Geometry check sheet. Reference: drawing and pictorial views, mm from the part's lowest x, y, z. Coordinates: 2 decimals unless noted, no trailing zeros. Write each loop counter-clockwise with the first axis right and the second up, starting at its lowest first coordinate (ties: lowest second). Pieces come first, ordered by that corner, then holes. Notation, with made-up numbers: (-28.5, 3.5) - (-14.5, 3.5) arc R21 ccw to (-14.5, 26.5) - close; hole circle Ø9 at (36, 77). An arc over 180 degrees is marked (long way). Use one line per item in the form item = value. Start each with the question number.
(1) Sectioned sample at B-B (x = 58.42). Record the cut outline in (y, z).
(2) Sectioned sample at A-A (y = 6.35). Record the cut outline in (x, z) (3 decimals).
(3) Material ranges on line 1 (Z direction, x = 12.7, y = 9) (3 decimals); line 2 (Y direction, x = 58.42, z = 9.5); line 3 (X direction, y = 7.25, z = 13), recorded low to high. Write a range as [from, to].
(4) Mould release check, pull along X, two halves, no side actions. Record for the marked faces 1, 2, 3 and 4: released by +X, released by -X, zero draft, split by the parting line, or undercut.
(5) Sectioned sample at C-C (z = 15.75). Record the cut outline in (x, y).
(6) Gauge pin test, flat end, axial feed: pin 1 Ø1 at (x, z) = (46.5, 16) entering from -Y. Record the tip position at first contact, or that the pin passes through.
(7) Sectioned sample at D-D (y = 1). Record the cut outline in (x, z) (3 decimals).
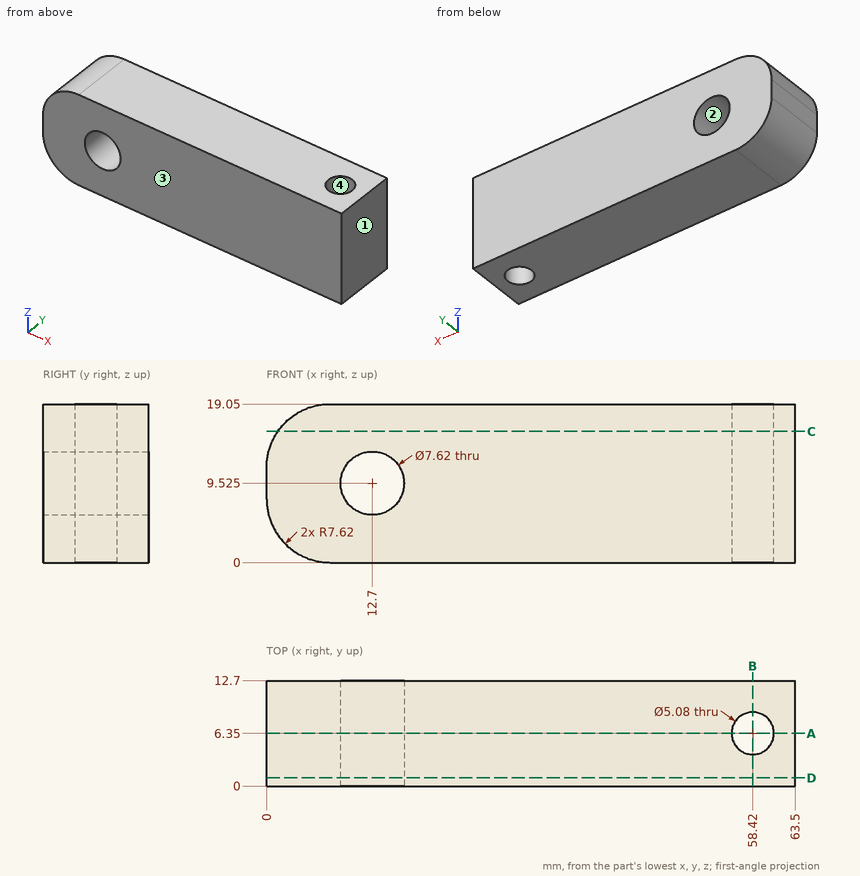
Answers below:
q1.outline = (0, 0) - (3.81, 0) - (3.81, 19.05) - (0, 19.05) - close; (8.89, 0) - (12.7, 0) - (12.7, 19.05) - (8.89, 19.05) - close
q2.outline = (0, 7.62) arc R7.62 ccw to (7.62, 0) - (55.88, 0) - (55.88, 19.05) - (7.62, 19.05) arc R7.62 ccw to (0, 11.43) - close; (60.96, 0) - (63.5, 0) - (63.5, 19.05) - (60.96, 19.05) - close; hole circle Ø7.62 at (12.7, 9.525)
q3.line_1 = [0, 5.715], [13.335, 19.05]
q3.line_2 = [0, 3.81], [8.89, 12.7]
q3.line_3 = [0.16, 11.14], [14.26, 56.04], [60.8, 63.5]
q4.face_1 = released by +X
q4.face_2 = undercut
q4.face_3 = zero draft
q4.face_4 = undercut
q5.outline = (1.34, 0) - (63.5, 0) - (63.5, 12.7) - (1.34, 12.7) - close; hole circle Ø5.08 at (58.42, 6.35)
q6.pin_1 = 0
q7.outline = (0, 7.62) arc R7.62 ccw to (7.62, 0) - (63.5, 0) - (63.5, 19.05) - (7.62, 19.05) arc R7.62 ccw to (0, 11.43) - close; hole circle Ø7.62 at (12.7, 9.525)
